```python
from build123d import *

# Parameters (mm, degrees)
F0_W     = 5
F0_H     = 40
F1_DEPTH = 80
F3_DEPTH = 25


with BuildPart() as f1:
    # F0 (on Front) → F1 (new body)
    with BuildSketch(Plane.XZ):
        with Locations((-15.079972, -4.429811)):
            Rectangle(F0_W, F0_H)
        Polygon((-12.579972, -24.429811), (-17.579972, -24.429811), (-17.579972, -29.429809), (42.420028, -29.429809), (42.420028, -24.429811), (37.420028, -24.429811), align=None)
        Polygon((-22.579972, 15.570189), (-17.579972, 15.570189), (-12.579972, 15.570189), (-7.579972, 15.570189), (-7.579972, 20.570189), (-22.579972, 20.570189), align=None)
        with Locations((39.920028, -4.429811)):
            Rectangle(F0_W, F0_H)
        Polygon((32.420028, 15.570189), (37.420028, 15.570189), (42.420028, 15.570189), (47.420028, 15.570189), (47.420028, 20.570189), (32.420028, 20.570189), align=None)
    extrude(amount=F1_DEPTH)

    # F2 (on face) → F3 (cut)
    with BuildSketch(Plane(origin=(0, 0, -29.429809), x_dir=(1, 0, 0), z_dir=(0, 0, -1))):
        with BuildLine():
            ThreePointArc((17.420028, 65), (12.420028, 70), (7.420028, 65))
            Line((7.420028, 65), (7.420028, 15))
            ThreePointArc((7.420028, 15), (12.420028, 10), (17.420028, 15))
            Line((17.420028, 15), (17.420028, 65))
        make_face()
    extrude(amount=-F3_DEPTH, mode=Mode.SUBTRACT)


solid = f1.part
```
For this review, take the finished solid that the model builds, in its own axes (mm). A direction names the side the tool comes from. Coordinates: 2 decimals unless noted, no trailing zeros. Write each loop counter-clockwise with the first axis right and the second up, starting at its lowest first coordinate (ties: lowest second). Pieces come first, ordered by that corner, then holes. Notation, with made-up numbers: (78.5, -5) -> (111.5, -5) arc R19 ccw to (111.5, 10) -> close; hole circle Ø3 at (36.5, -5.5). An arc over 180 degrees is marked (long way). Put each result on its own line as item: value.
Q1. The part is to be moulded in two halves that separate along Y. For faces 4 (the flat face through (12, -80, -25)), 5 (the flat face through (7.42, -40, -27)), 6 (the cylindrical face through (12.3, -10, -27)), 7 (the flat face through (-15, -39, 20.57)), say which applies: +Y half, -Y half, draft (parallel to the pull), parting line (faces both ways), or undercut.
From the geometry:
face 4: -Y half
face 5: undercut
face 6: undercut
face 7: draft
Q2. Wall thickness on L1, parallel to X at y = -7, z = 8; L2, parallel to Z at x = 30, y = -52; L3, parallel to X at y = -27.5, z = -25.5: over which ranges is each line inside the solid? List them lowest first.
From the geometry:
L1: x = -17.58 to -12.58, 37.42 to 42.42
L2: z = -29.43 to -24.43
L3: x = -17.58 to 7.42, 17.42 to 42.42
Q3. Tool access review of faces 1 (the flat face through (35, -39, 15.57)), 2 (the flat face through (-17.58, -39, -7)), 3 (the flat face through (-7.58, -39, 18)): name each direction out of +Z, -Z, +X, -X, +Y, -Y from which nothing blocks a thin tool from reaching the whole face with its end or side.
From the geometry:
face 1: +Y, -Y
face 2: -Z, -X, +Y, -Y
face 3: +Z, +Y, -Y
Q4. Take a section at B-B, the plane z = 17.5. State the section outline as (x, y) points, then the cut area to 3 significant figures.
From the geometry:
outline: (-22.58, -80) -> (-7.58, -80) -> (-7.58, 0) -> (-22.58, 0) -> close; (32.42, -80) -> (47.42, -80) -> (47.42, 0) -> (32.42, 0) -> close
area: 2,400 mm2
Q5. Take a section at C-C, the plane z = -13. State the section outline as (x, y) points, then the cut area to 3 significant figures.
From the geometry:
outline: (-17.58, -80) -> (-12.58, -80) -> (-12.58, 0) -> (-17.58, 0) -> close; (37.42, -80) -> (42.42, -80) -> (42.42, 0) -> (37.42, 0) -> close
area: 800 mm2
Q6. Take a section at A-A, the plane y = -57. State the section outline as (x, z) points, then the cut area to 3 significant figures.
From the geometry:
outline: (-22.58, 15.57) -> (-17.58, 15.57) -> (-17.58, -29.43) -> (7.42, -29.43) -> (7.42, -24.43) -> (-12.58, -24.43) -> (-12.58, 15.57) -> (-7.58, 15.57) -> (-7.58, 20.57) -> (-22.58, 20.57) -> close; (17.42, -29.43) -> (42.42, -29.43) -> (42.42, 15.57) -> (47.42, 15.57) -> (47.42, 20.57) -> (32.42, 20.57) -> (32.42, 15.57) -> (37.42, 15.57) -> (37.42, -24.43) -> (17.42, -24.43) -> close
area: 800 mm2
Q7. Clearance check with flat-ended pins moving along their axes: pin 1 Ø10 at (y, z) = (-72, -22.5) entering from +X; pin 2 Ø10 at (y, z) = (-23, 5.5) entering from -X; pin 3 Ø8 at (x, z) = (-10, -1.5) entering from +Y; pin 4 Ø2.5 at (x, y) = (-20, -25.5) entering from -Z. State where each tip first meets the part, or that it passes through.
From the geometry:
pin 1: stops at x = 42.42
pin 2: stops at x = -17.58
pin 3: stops at y = 0
pin 4: stops at z = 15.57
Q8. Take a section at D-D, the plane y = -11. State the section outline as (x, z) points.
From the geometry:
outline: (-22.58, 15.57) -> (-17.58, 15.57) -> (-17.58, -29.43) -> (9.42, -29.43) -> (9.42, -24.43) -> (-12.58, -24.43) -> (-12.58, 15.57) -> (-7.58, 15.57) -> (-7.58, 20.57) -> (-22.58, 20.57) -> close; (15.42, -29.43) -> (42.42, -29.43) -> (42.42, 15.57) -> (47.42, 15.57) -> (47.42, 20.57) -> (32.42, 20.57) -> (32.42, 15.57) -> (37.42, 15.57) -> (37.42, -24.43) -> (15.42, -24.43) -> close
